Can you work these out from the model? Positions are in its coordinate system, mm. Face numbers are marked on the shaded views. A direction names the side the tool comes from. Coordinates: 2 decimals unless noted, no trailing zeros. Loops run counter-clockwise (first coordinate to the right, second up) from the corner with the lowest first, then second, coordinate; pieces in that order, holes last.
```python
from build123d import *

# Parameters (mm, degrees)
F0_R     = 2.5
F1_DEPTH = 20
F2_R     = 4.99999
F3_R     = 2


# Not quite as in the source:
# - a fillet or chamfer is up to 0.001 mm smaller than in the source, because OpenCascade refuses the exact size


with BuildPart() as f1:
    # F0 (on Front) → F1 (new body)
    with BuildSketch(Plane.XZ):
        Polygon((22.5, 10.5), (-22.5, 10.5), (-22.5, -10.5), (-12.5, -10.5), (-12.5, 0.5), (12.5, 0.5), (12.5, -10.5), (22.5, -10.5), align=None)
        with Locations((-17.5, -6.5)):
            Circle(F0_R, mode=Mode.SUBTRACT)
        with Locations((17.5, -6.5)):
            Circle(F0_R, mode=Mode.SUBTRACT)
    extrude(amount=F1_DEPTH)

    # F2 (radius 5 in the source; OpenCascade refuses exactly that, so slightly less here)
    f2_edges = [f1.edges().sort_by_distance(p)[0] for p in [
        (-22.5, -10, -10.5),
        (-12.5, -10, -10.5),
        (12.5, -10, -10.5),
        (22.5, -10, -10.5),
    ]]
    fillet(f2_edges, radius=F2_R)

    # F3
    f3_edges = [f1.edges().sort_by_distance(p)[0] for p in [
        (22.5, -10, 10.5),
        (-22.5, -10, 10.5),
    ]]
    fillet(f3_edges, radius=F3_R)


solid = f1.part
```
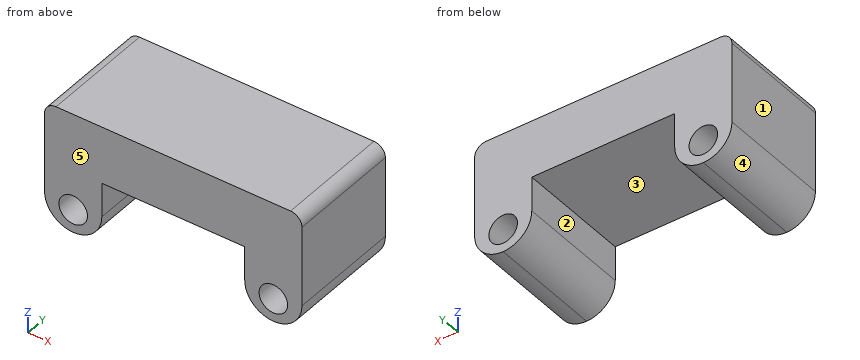
Item 1: We'd pull the mould along X, two halves only. Please class the marked faces 3, 4 and 5: +X half, -X half, draft (parallel to the pull), parting line (faces both ways), or undercut.
Results are:
face 3: undercut
face 4: -X half
face 5: draft
Item 2: On a 3-axis mill with a long thin cutter (end or side, diameter ignored), from which of +Z, -Z, +X, -X, +Y, -Y can I reach the whole of each face in a straight line? I mean the marked faces 1 and 2. Say none if no direction works.
Results are:
face 1: +Z, -Z, -X, +Y, -Y
face 2: -Z, +Y, -Y
Item 3: Suppose I cut it at A-A, the plane z = -2.25. Please give me the cut outline in (x, y), plus the area to 3 significant figures.
Results are:
outline: (-22.5, -20) - (-12.5, -20) - (-12.5, 0) - (-22.5, 0) - close; (12.5, -20) - (22.5, -20) - (22.5, 0) - (12.5, 0) - close
area: 400 mm2
Item 4: Suppose I cut it at D-D, the plane x = 19. Please give me the cut outline in (y, z).
Results are:
outline: (-20, -10.27) - (0, -10.27) - (0, -8.5) - (-20, -8.5) - close; (-20, -4.5) - (0, -4.5) - (0, 10.5) - (-20, 10.5) - close
Item 5: I'm going to push flat-ended pins straight in: P1, Ø1.5, axis at x = -12, z = 4.5, coming from the +Y side; P2, Ø6, axis at x = -0.5, y = -7, coming from the -Z side. Where does each tip first touch, or does it pass through?
Results are:
P1: stops at y = 0
P2: stops at z = 0.5
Item 6: I need wall thicknesses on line 1 along X through (y, z) = (-6.25, -1.5); line 2 along Z through (x, y) = (-17.5, -4.75); line 3 along X through (y, z) = (-18.5, -6). Which ranges of each line are inside material? Lowest first, please.
Results are:
line 1: x = -22.5 to -12.5, 12.5 to 22.5
line 2: z = -10.5 to -9, -4 to 10.5
line 3: x = -22.47 to -19.95, -15.05 to -12.53, 12.53 to 15.05, 19.95 to 22.47
Item 7: Suppose I cut it at C-C, the plane z = -6.5. Please give me the cut outline in (x, y).
Results are:
outline: (-22.4, -20) - (-20, -20) - (-20, 0) - (-22.4, 0) - close; (-15, -20) - (-12.6, -20) - (-12.6, 0) - (-15, 0) - close; (12.6, -20) - (15, -20) - (15, 0) - (12.6, 0) - close; (20, -20) - (22.4, -20) - (22.4, 0) - (20, 0) - close
Item 8: Suppose I cut it at B-B, the plane y = -4. Count the separate pieces of the cut face and the enclosed holes in it, plus the area to 3 significant figures.
Results are:
separate pieces: 1
enclosed holes: 2
area: 608 mm2
